Read the model definition and answer for the solid it produces. Units are mm, in the model's axes. A direction names the side the tool comes from. Round coordinates to 2 decimals unless told otherwise and drop trailing zeros. Write each loop counter-clockwise with the first axis right and the second up, starting at its lowest first coordinate (ties: lowest second). Pieces come first, ordered by that corner, then holes. Notation, with made-up numbers: (20.5, -7.5) - (54.5, -7.5) arc R18 ccw to (54.5, 14.5) - close; hole circle Ø11 at (-1.75, 22). An arc over 180 degrees is marked (long way). One line per item, written item: value. Start each with the question number.
(1) The mould has two halves that part along Y. Classify faces 1 (the face through (-1.73, 10.74, 7.81)), 2 (the face through (-6, 5, 0)), 3 (the face through (-2, 10, -6)), 4 (the face through (3, 12, 3)): +Y half, -Y half, draft (parallel to the pull), parting line (faces both ways), or undercut.
(2) A flat-ended cylindrical pin translates along its axis: pin 1 Ø1.5 at (x, y) = (-2, 10) entering from -Z. Find the tip coordinate at first contact, or state that the pin passes through.
(3) A cutting plane is placed at B-B, the plane z = 0. Determine the outline of the cut face in (x, y), plus the area to 3 significant figures.
(4) For faces 5 (the face through (-1.73, -0.74, 7.81)), 6 (the face through (-2, 0, -6)), determine the directions among +Z, -Z, +X, -X, +Y, -Y from which every point of the face is accessible in a straight line to the end or side of a thin tool.
(5) A cutting plane is placed at A-A, the plane x = 0. Determine the outline of the cut face in (y, z), plus the area to 3 significant figures.
(6) Find the intervals of material crossed by L1, parallel to Y at x = 3.5, z = 5.25; L2, parallel to Z at x = 0, y = 2.5, in increasing order.
(7) A cutting plane is placed at C-C, the plane y = 4.75. Determine the outline of the cut face in (x, z).
from build123d import *

# Parameters (mm, degrees)
SKETCH1_R                = 6
SKETCH1_R_2              = 4
BOSS_EXTRUDE1_DEPTH      = 12
BOSS_EXTRUDE1_DEPTH_BACK = 2
SKETCH1_3_R              = 8
SKETCH1_3_R_2            = 6
BOSS_EXTRUDE2_DEPTH      = 2
BOSS_EXTRUDE3_START      = 10
SKETCH1_4_R              = 8
SKETCH1_4_R_2            = 6
BOSS_EXTRUDE3_DEPTH      = 2
CHAMFER1_SIZE            = 0.5


with BuildPart() as part:
    # Sketch1 → Boss-Extrude1 (new body, two sides)
    with BuildSketch(Plane(origin=(0, 0, 0), x_dir=(1, 0, 0), z_dir=(0, 1, 0))) as boss_extrude1_sk:
        Circle(SKETCH1_R)
        Circle(SKETCH1_R_2, mode=Mode.SUBTRACT)
    extrude(amount=BOSS_EXTRUDE1_DEPTH)
    extrude(boss_extrude1_sk.sketch, amount=-BOSS_EXTRUDE1_DEPTH_BACK)

    # Sketch1_3 → Boss-Extrude2 (add)
    with BuildSketch(Plane(origin=(0, 0, 0), x_dir=(1, 0, 0), z_dir=(0, 1, 0))):
        Circle(SKETCH1_3_R)
        Circle(SKETCH1_3_R_2, mode=Mode.SUBTRACT)
    extrude(amount=-BOSS_EXTRUDE2_DEPTH)

    # Sketch1_4 → Boss-Extrude3 (add)
    with BuildSketch(Plane(origin=(0, 0, 0), x_dir=(1, 0, 0), z_dir=(0, 1, 0)).offset(BOSS_EXTRUDE3_START)):
        Circle(SKETCH1_4_R)
        Circle(SKETCH1_4_R_2, mode=Mode.SUBTRACT)
    extrude(amount=BOSS_EXTRUDE3_DEPTH)

    # Chamfer1
    chamfer1_edges = [part.edges().sort_by_distance(p)[0] for p in [
        (-8, -2, 0),
        (-8, 12, 0),
    ]]
    chamfer(chamfer1_edges, length=CHAMFER1_SIZE)


solid = part.part
Here are the results:
1. face 1: draft
1. face 2: undercut
1. face 3: undercut
1. face 4: +Y half
2. pin 1: z = -7.9
3. outline: (-8, -1.5) - (-7.5, -2) - (-4, -2) - (-4, 12) - (-7.5, 12) - (-8, 11.5) - (-8, 10) - (-6, 10) - (-6, 0) - (-8, 0) - close; (4, -2) - (7.5, -2) - (8, -1.5) - (8, 0) - (6, 0) - (6, 10) - (8, 10) - (8, 11.5) - (7.5, 12) - (4, 12) - close
3. area: 71.5 mm²
4. face 5: +Y, -Y
4. face 6: none
5. outline: (-2, -7.5) - (-1.5, -8) - (0, -8) - (0, -6) - (10, -6) - (10, -8) - (11.5, -8) - (12, -7.5) - (12, -4) - (-2, -4) - close; (-2, 4) - (12, 4) - (12, 7.5) - (11.5, 8) - (10, 8) - (10, 6) - (0, 6) - (0, 8) - (-1.5, 8) - (-2, 7.5) - close
5. area: 71.5 mm²
6. L1: -2 to 0, 10 to 12
6. L2: -6 to -4, 4 to 6
7. outline: circle Ø12 at (0, 0); hole circle Ø8 at (0, 0)
